```python
from build123d import *

# Parameters (mm, degrees)
SKETCH1_W                       = 20
SKETCH1_H                       = 22.5
BOSS_EXTRUDE1_DEPTH             = 10
CBORE_FOR_M2_SHCS1_D            = 2.4
CBORE_FOR_M2_SHCS1_CBORE_D      = 4.4
CBORE_FOR_M2_SHCS1_CBORE_DEPTH  = 4
SKETCH4_W                       = 24
SKETCH4_H                       = 12
BOSS_EXTRUDE2_DEPTH             = 12.5
TAP_DRILL_FOR_M3X0_5_TAP1_D     = 2.5
TAP_DRILL_FOR_M3X0_5_TAP1_DEPTH = 4
TAP_DRILL_FOR_M3X0_5_TAP1_TIP   = 0.751075774
TAP_DRILL_FOR_M3X0_5_TAP2_D     = 2.5
TAP_DRILL_FOR_M3X0_5_TAP2_DEPTH = 4
TAP_DRILL_FOR_M3X0_5_TAP2_TIP   = 0.751075774
CUT_EXTRUDE1_DEPTH              = 1


with BuildPart() as part:
    # Sketch1 → Boss-Extrude1 (new body)
    with BuildSketch(Plane.XY):
        with Locations((10, 11.25)):
            Rectangle(SKETCH1_W, SKETCH1_H)
    extrude(amount=BOSS_EXTRUDE1_DEPTH)

    # CBORE for M2 SHCS1 (through all)
    with Locations(Plane.XY.offset(10)):
        with Locations((4, 15.25), (16, 15.25), (16, 7.25), (4, 7.25)):
            CounterBoreHole(CBORE_FOR_M2_SHCS1_D / 2, CBORE_FOR_M2_SHCS1_CBORE_D / 2, CBORE_FOR_M2_SHCS1_CBORE_DEPTH)

    # Sketch4 → Boss-Extrude2 (add)
    with BuildSketch(Plane(origin=(0, 22.5, 0), x_dir=(1, 0, 0), z_dir=(0, 1, 0))):
        with Locations((10, -4)):
            Rectangle(SKETCH4_W, SKETCH4_H)
    extrude(amount=BOSS_EXTRUDE2_DEPTH)

    # Tap Drill for M3x0.5 Tap1
    with Locations(Plane(origin=(20, 0, 0), x_dir=(0, 0, -1), z_dir=(1, 0, 0))):
        with Locations((-4.751843682, 18.25), (-4.751843682, 4.25)):
            Hole(TAP_DRILL_FOR_M3X0_5_TAP1_D / 2, depth=TAP_DRILL_FOR_M3X0_5_TAP1_DEPTH)
            with Locations((0, 0, -(TAP_DRILL_FOR_M3X0_5_TAP1_DEPTH + TAP_DRILL_FOR_M3X0_5_TAP1_TIP / 2))):  # 118° drill point
                Cone(0, TAP_DRILL_FOR_M3X0_5_TAP1_D / 2, TAP_DRILL_FOR_M3X0_5_TAP1_TIP, mode=Mode.SUBTRACT)

    # Tap Drill for M3x0.5 Tap2
    with Locations(Plane.ZY):
        with Locations((4.751843682, 18.25), (4.751843682, 4.25)):
            Hole(TAP_DRILL_FOR_M3X0_5_TAP2_D / 2, depth=TAP_DRILL_FOR_M3X0_5_TAP2_DEPTH)
            with Locations((0, 0, -(TAP_DRILL_FOR_M3X0_5_TAP2_DEPTH + TAP_DRILL_FOR_M3X0_5_TAP2_TIP / 2))):  # 118° drill point
                Cone(0, TAP_DRILL_FOR_M3X0_5_TAP2_D / 2, TAP_DRILL_FOR_M3X0_5_TAP2_TIP, mode=Mode.SUBTRACT)

    # Sketch9 → Cut-Extrude1 (cut)
    with BuildSketch(Plane.XZ.offset(-22.5)):
        Polygon((0, 0), (0, 10), (-2, 10), (-2, -2), (22, -2), (22, 10), (20, 10), (20, 0), align=None)
    extrude(amount=-CUT_EXTRUDE1_DEPTH, mode=Mode.SUBTRACT)


solid = part.part
```
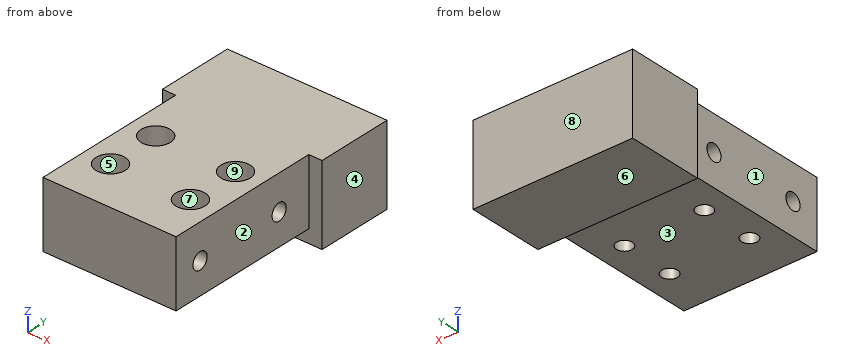
Can you work these out from the model? Positions are in its coordinate system, mm. Face numbers are marked on the shaded views. A direction names the side the tool comes from. Coordinates: 2 decimals unless noted, no trailing zeros. Write each loop counter-clockwise with the first axis right and the second up, starting at its lowest first coordinate (ties: lowest second). Pieces come first, ordered by that corner, then holes. Notation, with made-up numbers: M 39,-20.75 L 57,-20.75 A9 cw 57,-8.75 Z; hole C 57.5,46 d9. An arc over 180 degrees is marked long. Answer as CSV lines item,"result".
Item 1: We'd pull the mould along Y, two halves only. Please class the marked faces 6, 7, 8 and 9: +Y half, -Y half, draft (parallel to the pull), parting line (faces both ways), or undercut.
Geometry results:
face 6,"draft"
face 7,"undercut"
face 8,"+Y half"
face 9,"undercut"
Item 2: Please list where these lines run through material, in increasing order: line 1 along X through (y, z) = (6.5, 1.5); line 2 along Z through (x, y) = (19.2, 4.25); line 3 along X through (y, z) = (7, 4.5).
Geometry results:
line 1,"x = 0 to 3.06, 4.94 to 15.06, 16.94 to 20"
line 2,"z = 0 to 3.5, 6 to 10"
line 3,"x = 0 to 2.83, 5.17 to 14.83, 17.17 to 20"
Item 3: Imagine slicing it at C-C on y = 7.25. List the corners of the cut face in (x, z) for me, plus the area to 3 significant figures.
Geometry results:
outline,"M 0,0 L 2.8,0 L 2.8,6 L 1.8,6 L 1.8,10 L 0,10 Z; M 5.2,0 L 14.8,0 L 14.8,6 L 13.8,6 L 13.8,10 L 6.2,10 L 6.2,6 L 5.2,6 Z; M 17.2,0 L 20,0 L 20,10 L 18.2,10 L 18.2,6 L 17.2,6 Z"
area,"136 mm2"
Item 4: Imagine slicing it at B-B on x = 16.5. List the corners of the cut face in (y, z) for me.
Geometry results:
outline,"M 0,0 L 6.16,0 L 6.16,6 L 5.11,6 L 5.11,10 L 0,10 Z; M 8.34,0 L 14.16,0 L 14.16,6 L 13.11,6 L 13.11,10 L 9.39,10 L 9.39,6 L 8.34,6 Z; M 16.34,0 L 23.5,0 L 23.5,-2 L 35,-2 L 35,10 L 17.39,10 L 17.39,6 L 16.34,6 Z; hole C 4.25,4.75 d2.5; hole C 18.25,4.75 d2.5"
Item 5: Imagine slicing it at A-A on z = 1.75. List the corners of the cut face in (x, y) for me, plus the area to 3 significant figures.
Geometry results:
outline,"M -2,23.5 L 0,23.5 L 0,0 L 20,0 L 20,23.5 L 22,23.5 L 22,35 L -2,35 Z; hole C 4,7.25 d2.4; hole C 4,15.25 d2.4; hole C 16,7.25 d2.4; hole C 16,15.25 d2.4"
area,"728 mm2"
Item 6: Imagine slicing it at D-D on x = 12.5. List the corners of the cut face in (y, z) for me, plus the area to 3 significant figures.
Geometry results:
outline,"M 0,0 L 23.5,0 L 23.5,-2 L 35,-2 L 35,10 L 0,10 Z"
area,"373 mm2"
Item 7: On a 3-axis mill with a long thin cutter (end or side, diameter ignored), from which of +Z, -Z, +X, -X, +Y, -Y can I reach the whole of each face in a straight line? I mean the marked faces 1, 2, 3, 4 and 5. Say none if no direction works.
Geometry results:
face 1,"+Z, -Z, -X, -Y"
face 2,"+Z, -Z, +X, -Y"
face 3,"-Z, +X, -X, -Y"
face 4,"+Z, -Z, +X, +Y, -Y"
face 5,"+Z"
Item 8: I'm going to push flat-ended pins straight in: P1, Ø4, axis at y = 18.25, z = 4.75, coming from the -X side; P2, Ø10, axis at x = 10, y = 13.5, coming from the -Z side; P3, Ø5, axis at y = 17, z = 4, coming from the +X side; P4, Ø1.4, axis at x = 4, y = 7.25, coming from the -Z side. Where does each tip first touch, or does it pass through?
Geometry results:
P1,"stops at x = 0"
P2,"stops at z = 0"
P3,"stops at x = 20"
P4,"passes through"
